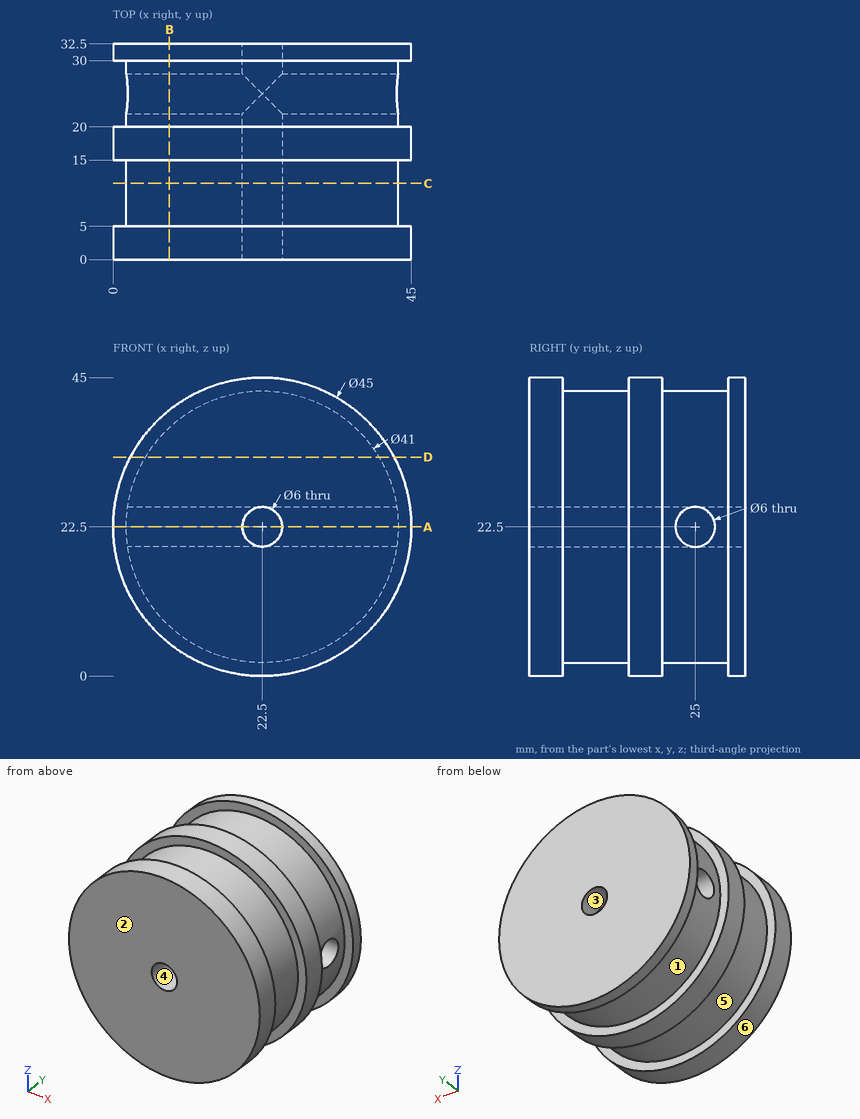
Source: three-view drawing plus pictorial views. Frame: mm from the lowest corner of the part. A direction names the side the tool comes from. Give positions to 0.01 mm unless a question says otherwise; leave off trailing zeros. Order: outer loops, then holes, each group sorted by start corner. A loop starts at its lowest first (then second) coordinate and runs counter-clockwise, first axis right, second up. Notation, with made-up numbers: M 27.5,47.25 L 68.5,47.25 A21 cw 68.5,58.25 Z; hole C 1,51 d7. An arc over 180 degrees is marked long. Return JSON: item names as keys, results as strings.
1) Section query C-C on y = 11.5. Output: boundary loops of the cut face in (x, z), and give its area (3 significant figures).
Taken from the geometry:
{"outline": "C 22.5,22.5 d41; hole C 22.5,22.5 d6", "area": "1,290 mm2"}
2) Access query for the marked faces 5 and 6. Directions: +Z, -Z, +X, -X, +Y, -Y. A direction counts if a zero-diameter tool reaches every point of the face in a straight line with its end or side. Return the directions, or none.
Taken from the geometry:
{"face 5": "none", "face 6": "+Y, -Y"}
3) Section query D-D on z = 33. Output: boundary loops of the cut face in (x, y).
Taken from the geometry:
{"outline": "M 2.6,0 L 42.4,0 L 42.4,5 L 40.11,5 L 40.11,15 L 42.4,15 L 42.4,20 L 40.11,20 L 40.11,30 L 42.4,30 L 42.4,32.5 L 2.6,32.5 L 2.6,30 L 4.89,30 L 4.89,20 L 2.6,20 L 2.6,15 L 4.89,15 L 4.89,5 L 2.6,5 Z"}
4) Section query B-B on x = 8.5. Output: boundary loops of the cut face in (y, z).
Taken from the geometry:
{"outline": "M 0,4.89 L 5,4.89 L 5,7.53 L 15,7.53 L 15,4.89 L 20,4.89 L 20,7.53 L 30,7.53 L 30,4.89 L 32.5,4.89 L 32.5,40.11 L 30,40.11 L 30,37.47 L 20,37.47 L 20,40.11 L 15,40.11 L 15,37.47 L 5,37.47 L 5,40.11 L 0,40.11 Z; hole C 25,22.5 d6"}
5) Section query A-A on z = 22.5. Count the separate pieces of the cut face and the enclosed holes in it, and give its area (4 significant figures).
Taken from the geometry:
{"separate pieces": "4", "enclosed holes": "0", "area": "977.5 mm2"}
6) Mould query, pull axis Z, two halves, no side actions, for the marked faces 1, 2, 3 and 4. Classes: released by +Z, released by -Z, zero draft, split by the parting line, or undercut.
Taken from the geometry:
{"face 1": "split by the parting line", "face 2": "zero draft", "face 3": "undercut", "face 4": "undercut"}
7) Contact query for flat-ended pins moving along their axis: pin 1 (2 mm diameter, centred on x = 37.5, y = 13, fed in from -Z) (3 decimals); pin 2 (8 mm diameter, centred on x = 29, z = 24.5, fed in from -Y); pin 3 (1.5 mm diameter, centred on x = 40, y = 9, fed in from +Z); pin 4 (8 mm diameter, centred on y = 25, z = 22.5, fed in from +X). Output: stop coordinate, or through.
Taken from the geometry:
{"pin 1": "stops at z = 7.525", "pin 2": "stops at y = 0", "pin 3": "stops at z = 34.32", "pin 4": "stops at x = 43"}
8) Line query: L1, parallel to Y at x = 27.25, z = 22.5; L2, parallel to Y at x = 2.5, z = 32; L3, parallel to Z at x = 27, y = 25. Output: solid intervals per line, ascending. Write a range as [from, to].
Taken from the geometry:
{"L1": "y = [0, 22], [28, 32.5]", "L2": "y = [0, 5], [15, 20], [30, 32.5]", "L3": "z = [2.5, 19.5], [25.5, 42.5]"}
